Could you check a few things on this model? Use its own coordinates, in mm. A direction names the side the tool comes from. Coordinates: 2 decimals unless noted, no trailing zeros. Loops run counter-clockwise (first coordinate to the right, second up) from the corner with the lowest first, then second, coordinate; pieces in that order, holes last. Notation, with made-up numbers: (53.5, 41) -> (61.5, 41) arc R22 cw to (61.5, 56) -> close; hole circle Ø4 at (-3.5, 8.5). An arc over 180 degrees is marked (long way). One line per question, with ' | ' between items.
```python
from build123d import *

# Parameters (mm, degrees)
SKETCH1_R           = 8.855
BOSS_EXTRUDE1_DEPTH = 5.045
SKETCH2_R           = 22.085
SKETCH2_R_2         = 8.855
BOSS_EXTRUDE2_DEPTH = 1.465
SKETCH4_R           = 24.49
SKETCH4_R_2         = 17.66
BOSS_EXTRUDE3_DEPTH = 2.66
BOSS_EXTRUDE4_START = 2.66
SKETCH5_R           = 24.49
SKETCH5_R_2         = 17.66
BOSS_EXTRUDE4_DEPTH = 2.66


with BuildPart() as part:
    # Sketch1 → Boss-Extrude1 (new, symmetric)
    with BuildSketch(Plane.XY):
        Circle(SKETCH1_R)
        with BuildLine():
            ThreePointArc((-1.226414925, 4.016952381), (0, -4.2), (1.226414925, 4.016952381))
            ThreePointArc((1.226414925, 4.016952381), (0, 2.96), (-1.226414925, 4.016952381))
        make_face(mode=Mode.SUBTRACT)
    extrude(amount=BOSS_EXTRUDE1_DEPTH, both=True)

    # Sketch2 → Boss-Extrude2 (add, symmetric)
    with BuildSketch(Plane.XY):
        with Locations(Location((0, 0, 0), (0, 0, 180))):
            Circle(SKETCH2_R)
        Circle(SKETCH2_R_2, mode=Mode.SUBTRACT)
    extrude(amount=BOSS_EXTRUDE2_DEPTH, both=True)

    # Sketch4 → Boss-Extrude3 (add)
    with BuildSketch(Plane.XY.offset(1.465)):
        Circle(SKETCH4_R)
        Circle(SKETCH4_R_2, mode=Mode.SUBTRACT)
    extrude(amount=BOSS_EXTRUDE3_DEPTH)

    # Sketch5 → Boss-Extrude4 (add)
    with BuildSketch(Plane(origin=(0, 0, -1.465), x_dir=(-1, 0, 0), z_dir=(0, 0, -1)).offset(BOSS_EXTRUDE4_START)):
        with Locations(Location((0, 0, 0), (0, 0, 180))):
            Circle(SKETCH5_R)
        with Locations(Location((0, 0, 0), (0, 0, 180))):
            Circle(SKETCH5_R_2, mode=Mode.SUBTRACT)
    extrude(amount=-BOSS_EXTRUDE4_DEPTH)


solid = part.part
```
Q1. For pin 1 (1.5 mm diameter, centred on x = 2, y = 17, fed in from -Z) (3 decimals); pin 2 (6 mm diameter, centred on y = -9, z = 3, fed in from -X); pin 3 (4 mm diameter, centred on x = 5.5, z = -1.5, fed in from +Y), each with a flat end and sliding along its axis, tell me the tip position at first contact or that it passes through.
Values follow:
pin 1: stops at z = -4.125 | pin 2: stops at x = -23.74 | pin 3: stops at y = 24.24
Q2. Imagine slicing it at D-D on y = -6. Write out the boundary of the cut face in (x, z) (1 decimal), plus the area to 3 significant figures.
Values follow:
outline: (-23.7, -4.1) -> (-16.6, -4.1) -> (-16.6, -1.5) -> (-6.5, -1.5) -> (-6.5, -5) -> (6.5, -5) -> (6.5, -1.5) -> (16.6, -1.5) -> (16.6, -4.1) -> (23.7, -4.1) -> (23.7, -1.5) -> (21.3, -1.5) -> (21.3, 1.5) -> (23.7, 1.5) -> (23.7, 4.1) -> (16.6, 4.1) -> (16.6, 1.5) -> (6.5, 1.5) -> (6.5, 5) -> (-6.5, 5) -> (-6.5, 1.5) -> (-16.6, 1.5) -> (-16.6, 4.1) -> (-23.7, 4.1) -> (-23.7, 1.5) -> (-21.3, 1.5) -> (-21.3, -1.5) -> (-23.7, -1.5) -> close | area: 294 mm2
Q3. We'd pull the mould along Y, two halves only. Please class faces 5 (the face through (-3.19, 24.28, 2.78)), 6 (the face through (-1.15, 8.78, -3.23)), 7 (the face through (-3.83, 17.24, -2.81)), 8 (the face through (16.2, -7.4, -4.125)): released by +Y, released by -Y, zero draft, split by the parting line, or undercut.
Values follow:
face 5: split by the parting line | face 6: undercut | face 7: undercut | face 8: zero draft
Q4. Please list where these lines run through material, in increasing order: L1, parallel to Z at x = 18, y = 13 (3 decimals); L2, parallel to X at y = -1, z = 3.75; L3, parallel to X at y = 7.5, z = -3.75. Write a range as [from, to].
Values follow:
L1: z = [-4.125, -1.465], [1.465, 4.125] | L2: x = [-24.47, -17.63], [-8.8, -4.08], [4.08, 8.8], [17.63, 24.47] | L3: x = [-23.31, -15.99], [-4.71, 4.71], [15.99, 23.31]
Q5. Imagine slicing it at C-C on z = 3.25. Write out the boundary of the cut face in (x, y) (3 decimals).
Values follow:
outline: circle Ø48.98 at (0, 0); circle Ø17.71 at (0, 0); hole circle Ø35.32 at (0, 0); hole (-1.226, 4.017) arc R4.2 ccw (long way) to (1.226, 4.017) arc R1.24 cw to start
Q6. For faces 1 (the face through (4.79, 21.56, 0.02)), 2 (the face through (8.1, -4.2, -1.465)), 3 (the face through (-1.15, 8.78, 3.28)), 4 (the face through (4, -2, -5.045)), which set-ups out of +Z, -Z, +X, -X, +Y, -Y let a thin tool reach every point of the face, with its end or its side?
Values follow:
face 1: none | face 2: -Z | face 3: +Z | face 4: -Z, +X, -X, +Y, -Y
